Check sheet for the drawn part. Datum: minimum x, y, z corner. Units: mm. Round coordinates to 2 decimals unless told otherwise and drop trailing zeros. Loops run counter-clockwise (first coordinate to the right, second up) from the corner with the lowest first, then second, coordinate; pieces in that order, holes last. Notation, with made-up numbers: (-9.75, -22) - (-5.75, -22) arc R31 cw to (-5.75, 12) - close; hole circle Ø8 at (10.5, 2.25). An arc over 180 degrees is marked (long way). Use CSV: the item, a comma, the result in double quotes.
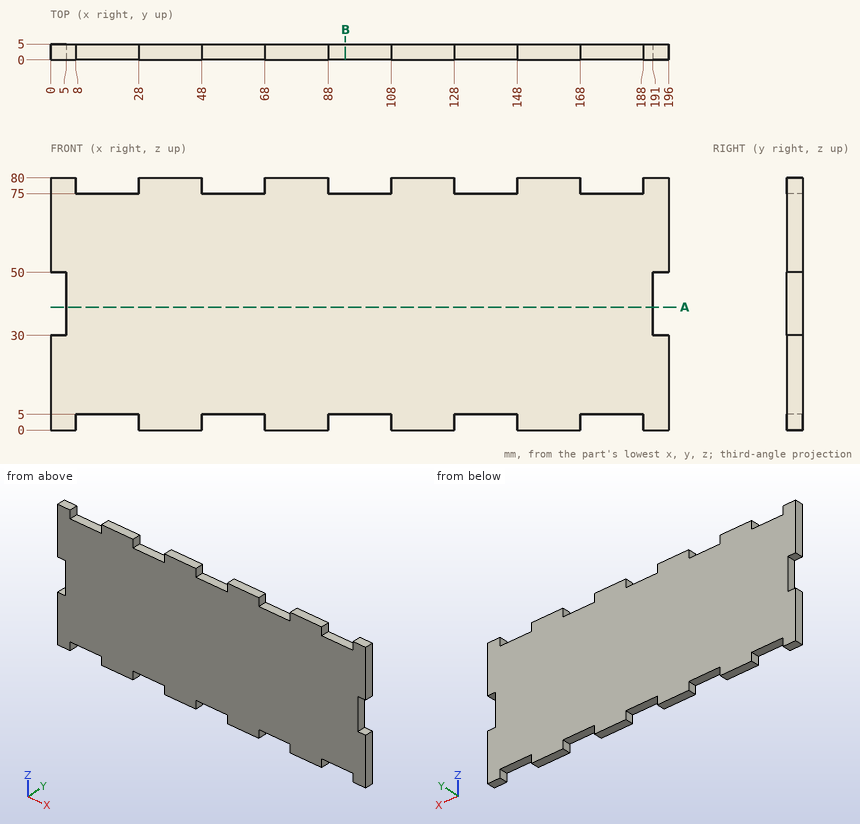
1) Gauge pin test, flat ends, axial feed: pin 1 Ø1.5 at (x, y) = (137.5, 4) entering from -Z; pin 2 Ø1.5 at (x, y) = (57.5, 2.5) entering from +Z. Record the tip position at first contact, or that the pin passes through.
Returned:
pin 1,"stops at z = 5"
pin 2,"stops at z = 75"
2) Cross-section at B-B, the plane x = 93.5. Record the cut outline in (y, z), then the cut area to 3 significant figures.
Returned:
outline,"(0, 5) - (5, 5) - (5, 75) - (0, 75) - close"
area,"350 mm²"
3) Cross-section at A-A, the plane z = 39. Record the cut outline in (x, y).
Returned:
outline,"(5, 0) - (191, 0) - (191, 5) - (5, 5) - close"
4) Thickness scan on probe 1 along X at (y, z) = (1.8, 77); probe 2 along Z at (x, y) = (63, 1.9); probe 3 along X at (y, z) = (1.3, 47.5). Record the ranges inside material, lowest first. Write a range as [from, to].
Returned:
probe 1,"x = [0, 8], [28, 48], [68, 88], [108, 128], [148, 168], [188, 196]"
probe 2,"z = [5, 75]"
probe 3,"x = [5, 191]"
